Autodesk Inventor part; units mm, degrees
ref_plane "YZ Plane" through (0, 0, 0) normal (1, 0, 0) x (0, 1, 0)
ref_plane "XZ Plane" through (0, 0, 0) normal (0, 1, 0) x (-1, 0, 0)
ref_plane "XY Plane" through (0, 0, 0) normal (0, 0, 1) x (1, 0, 0)
sketch "Sketch1" plane through (0, 0, 0) normal (1, 0, 0) x (0, 1, 0)
  line L0 (0, 0) -> (26.9875, 0)
  line L1 (26.9875, 0) -> (26.9875, -15.875)
  line L2 (26.9875, -15.875) -> (0, -15.875)
  line L3 (0, -15.875) -> (0, 0)
  line L4 (33.3375, -22.225) -> (33.3375, 6.35)
  line L5 (33.3375, 6.35) -> (-6.35, 6.35)
  line L6 (-6.35, 6.35) -> (-6.35, -22.225)
  line L7 (-6.35, -22.225) -> (33.3375, -22.225)
  dimension "d0" = 26.9875
  dimension "d1" = 15.875
  dimension "d2" = 6.35
extrude "Extrusion1" add sketch "Sketch1" along normal blind 101.6
sketch "Sketch2" plane through (0, -6.35, 6.35) normal (0, 0, 1) x (1, 0, 0)
  line L0 (0, 39.6875) -> (0, 0)
  line L1 (0, 19.8437) -> (101.6, 19.8437)
  line L2 (101.6, 39.6875) -> (101.6, 0)
  circle A0 centre (12.7, 19.8437) radius 6.35
  line L3 (50.8, 39.6875) -> (50.8, 0)
  line L4 (0, 0) -> (101.6, 0)
  circle A1 centre (88.9, 19.8437) radius 6.35
  line L5 (88.9, 26.1937) -> (12.7, 26.1937)
  line L6 (12.7, 13.4937) -> (88.9, 13.4937)
  point P0 (0, 6.35)
  dimension "d5" = 12.7
  dimension "d6" = 12.7
  dimension "d7" = 50.8
extrude "Extrusion2" cut sketch "Sketch2" against normal through all contours A0 L1 | L1 A0 | A0 L5 L3 L1 | L1 L3 L6 A0 | L3 L1 A1 L6 | L3 L5 A1 L1 | A1 L1 | A1 L1
fillet "Fillet1" radius 1.27 4 edges at (6.35, 13.4938, 6.35) (50.8, 19.8438, 6.35) (95.25, 13.4938, 6.35) (50.8, 7.1438, 6.35)
fillet "Fillet2" radius 1.27 4 edges at (50.8, 7.1438, 0) (95.25, 13.4938, 0) (50.8, 19.8438, 0) (6.35, 13.4938, 0)
properties part number "housing"
CAD build for the part. Positions are in the model's coordinates, mm. A direction names the side the tool comes from. Coordinates: 2 decimals unless noted, no trailing zeros. Order: outer loops, then holes, each group sorted by start corner. A loop starts at its lowest first (then second) coordinate and runs counter-clockwise, first axis right, second up. Notation, with made-up numbers: (38.5, 56) - (82.5, 56) arc R25 cw to (82.5, 83) - close; hole circle Ø9 at (77.5, -5). An arc over 180 degrees is marked (long way). Use a Markdown table: item, result. Add a question column.
(1) Pull direction X, two halves, no side cores. Call faces 4 (the face through (0, 13, 2)), 5 (the face through (50, 33.338, -8)), 6 (the face through (95.25, 13.35, -19.01)): +X half, -X half, draft (parallel to the pull), parting line (faces both ways), or undercut.
(2) Which spindle directions (+Z, -Z, +X, -X, +Y, -Y) get a long thin tool onto all of the face, cutting with end or side? Do faces 1 (the face through (95.25, 13.35, 3.2)), 2 (the face through (50, 26.988, -8)), 3 (the face through (50, 22, -22.225)). Say none if no direction does.
(3) Flat gauge pin, fed straight in: pin 1 (13.5 mm diameter, centred on x = 50.5, y = 13, fed in from +Z). Where does the tip first touch, or does it go through?
(4) Saw through at C-C (y = 22.5). Give the cut face in (x, z) (3 decimals).
(5) Saw through at D-D (y = 12). Count the separate pieces of the cut face and the enclosed holes in it, then the cut area to 3 significant figures.
(6) Drill centre lines: line 1 along Y through (x, z) = (19, 2); line 2 along Y through (x, z) = (68, -15); line 3 along Z through (x, y) = (22, 22.5) (3 decimals). Where is each one in solid material? Low to high. Write a range as [from, to].
(7) Saw through at B-B (z = -1.25). Give the cut face in (x, y), then the cut area to 3 significant figures.
Solved:
| question | item | result |
|---|---|---|
| 1 | face 4 | -X half |
| 1 | face 5 | draft |
| 1 | face 6 | undercut |
| 2 | face 1 | +Z, -Z |
| 2 | face 2 | +X, -X |
| 2 | face 3 | -Z, +X, -X, +Y, -Y |
| 3 | pin 1 | stops at z = 6.29 |
| 4 | outline | (0, -22.225) - (101.6, -22.225) - (101.6, -15.875) - (0, -15.875) - close; (0, 0) - (101.6, 0) - (101.6, 6.35) - (0, 6.35) - close |
| 5 | separate pieces | 4 |
| 5 | enclosed holes | 0 |
| 5 | area | 164 mm² |
| 6 | line 1 | y = [-6.35, 7.14], [19.84, 33.34] |
| 6 | line 2 | y = [-6.35, 0], [26.99, 33.34] |
| 6 | line 3 | z = [-22.225, -15.875], [0, 6.35] |
| 7 | outline | (0, -6.35) - (101.6, -6.35) - (101.6, 0) - (0, 0) - close; (0, 26.99) - (101.6, 26.99) - (101.6, 33.34) - (0, 33.34) - close |
| 7 | area | 1,290 mm² |
